```python
from build123d import *

# Parameters (mm, degrees)
SKETCH_1_W = 17
SKETCH_1_H = 76.85
FILLET_1_R = 3
FILLET_2_R = 1


with BuildPart() as part:
    # 草图1 → 旋转1 (revolve)
    with BuildSketch(Plane.XY):
        with Locations((-8.5, 38.425)):
            Rectangle(SKETCH_1_W, SKETCH_1_H)
        Polygon((0, -11), (0, 0), (-17, 0), (-22.35, 0), (-22.35, -11), align=None)
    revolve(axis=Axis((0, 76.85, 0), (0, -1, 0)))

    # 圆角1
    fillet_1_edges = [part.edges().sort_by_distance(p)[0] for p in [
        (22.35, -11, 0),
        (22.35, 0, 0),
    ]]
    fillet(fillet_1_edges, radius=FILLET_1_R)

    # 圆角2
    fillet_2_edges = [part.edges().sort_by_distance(p)[0] for p in [
        (17, 76.85, 0),
    ]]
    fillet(fillet_2_edges, radius=FILLET_2_R)


solid = part.part
```
The listing builds one solid part. Answer for the finished solid, in the listing's coordinates (mm). A direction names the side the tool comes from. Coordinates: 2 decimals unless noted, no trailing zeros. Loops run counter-clockwise (first coordinate to the right, second up) from the corner with the lowest first, then second, coordinate; pieces in that order, holes last. Notation, with made-up numbers: (31.25, 19.5) - (90.25, 19.5) arc R22 ccw to (90.25, 45.5) - close; hole circle Ø5 at (79.25, 10). An arc over 180 degrees is marked (long way). Write item = value, one per line.
1) Section C-C (y = 71) is taken. Determine the outline of the cut face in (x, z).
Responses:
outline = circle Ø34 at (0, 0)
2) Which of the six approach directions +Z, -Z, +X, -X, +Y, -Y give full straight-line access (tool end or side, diameter ignored) to faces 1 (the face through (1.34, 0, 17.11)), 2 (the face through (0, -11, 0))?
Responses:
face_1 = +Y
face_2 = +Z, -Z, +X, -X, -Y
3) Find the intervals of material crossed by line 1 along Y through (x, z) = (8.5, -16); line 2 along X through (y, z) = (52, 9); line 3 along Z through (x, y) = (-8.5, 19.5), in increasing order.
Responses:
line_1 = -11 to 0
line_2 = -14.42 to 14.42
line_3 = -14.72 to 14.72
4) Section B-B (x = 0) is taken. Determine the outline of the cut face in (y, z).
Responses:
outline = (-11, -19.35) arc R3 ccw to (-8, -22.35) - (-3, -22.35) arc R3 ccw to (0, -19.35) - (0, -17) - (75.85, -17) arc R1 ccw to (76.85, -16) - (76.85, 16) arc R1 ccw to (75.85, 17) - (0, 17) - (0, 19.35) arc R3 ccw to (-3, 22.35) - (-8, 22.35) arc R3 ccw to (-11, 19.35) - close
5) Each of these flat-tipped pins is pushed along its axis until it touches: P1, Ø5, axis at y = 27.5, z = -1.5, coming from the -X side; P2, Ø1, axis at y = 23.5, z = -16, coming from the +X side; P3, Ø2, axis at y = 60, z = 13.5, coming from the +X side. Where does it stop, or does it pass through?
Responses:
P1 = -17
P2 = 6.98
P3 = 11.52
6) Section D-D (y = -4) is taken. Determine the outline of the cut face in (x, z), plus the area to 3 significant figures.
Responses:
outline = circle Ø44.7 at (0, 0)
area = 1,570 mm^2
7) Section A-A (z = 0) is taken. Determine the outline of the cut face in (x, y), plus the area to 3 significant figures.
Responses:
outline = (-22.35, -8) arc R3 ccw to (-19.35, -11) - (19.35, -11) arc R3 ccw to (22.35, -8) - (22.35, -3) arc R3 ccw to (19.35, 0) - (17, 0) - (17, 75.85) arc R1 ccw to (16, 76.85) - (-16, 76.85) arc R1 ccw to (-17, 75.85) - (-17, 0) - (-19.35, 0) arc R3 ccw to (-22.35, -3) - close
area = 3,100 mm^2
